Source: three-view drawing plus pictorial views. Frame: mm from the lowest corner of the part. A direction names the side the tool comes from. Coordinates: 2 decimals unless noted, no trailing zeros. Order: outer loops, then holes, each group sorted by start corner. A loop starts at its lowest first (then second) coordinate and runs counter-clockwise, first axis right, second up. Notation, with made-up numbers: (85.5, -5.5) - (110.5, -5.5) arc R22 ccw to (110.5, 16.5) - close; hole circle Ø3 at (89, 74). An arc over 180 degrees is marked (long way). One line per question, with ' | ' between items.
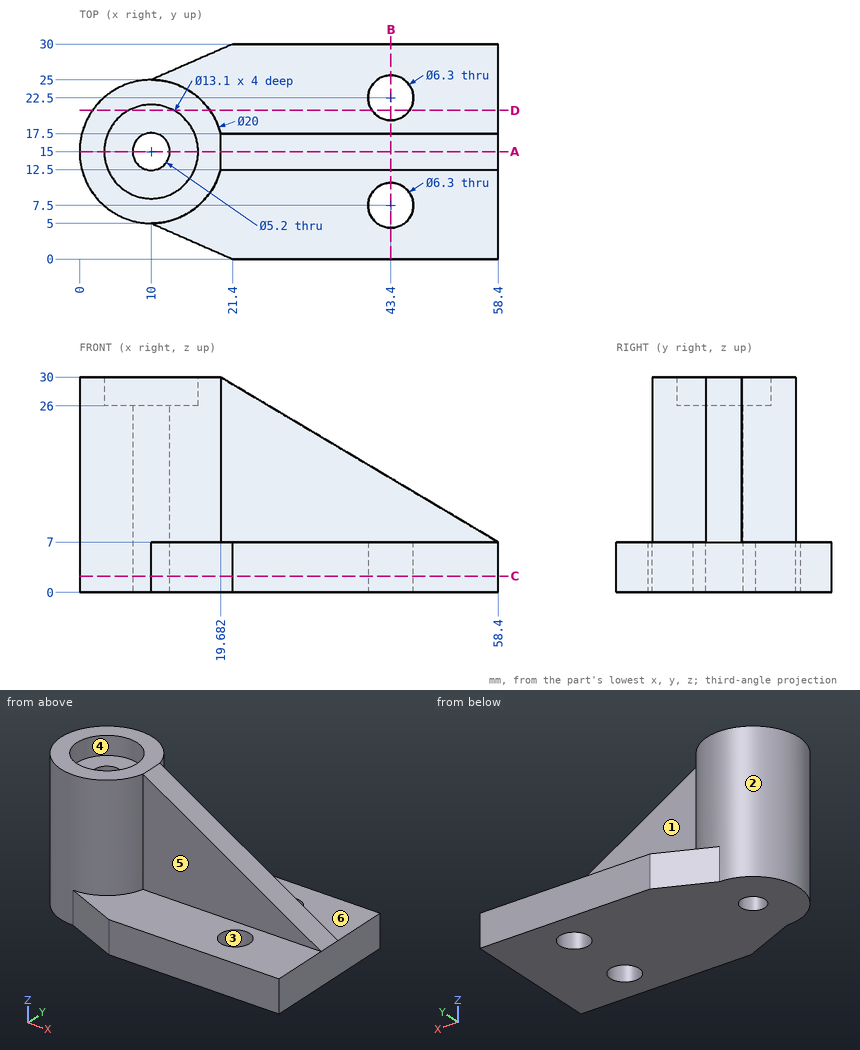
(1) Pull-direction query (X, two-part tool) for the marked faces 1, 2 and 3; classes: pulls with the +X half, pulls with the -X half, needs draft (parallel to the pull), parting line crosses it, or undercut.
Taken from the geometry:
face 1: needs draft | face 2: parting line crosses it | face 3: undercut
(2) Pin query (flat end, axial travel): P1, Ø1, axis at x = 29, y = 14, coming from the +Z side; P2, Ø5, axis at y = 21, z = 23.5, coming from the +X side; P3, Ø10, axis at x = 34, y = 3.5, coming from the +Z side. Return the tip coordinate at first contact, or that it passes through.
Taken from the geometry:
P1: stops at z = 24.76 | P2: stops at x = 19.37 | P3: stops at z = 7
(3) Cut plane A-A (y = 15). Return the cut outline in (x, z), and give its area (3 significant figures).
Taken from the geometry:
outline: (0, 0) - (7.4, 0) - (7.4, 26) - (3.45, 26) - (3.45, 30) - (0, 30) - close; (12.6, 0) - (58.4, 0) - (58.4, 7) - (19.68, 30) - (16.55, 30) - (16.55, 26) - (12.6, 26) - close | area: 1,120 mm²
(4) Material intervals for L1, parallel to Y at x = 43.4, z = 4; L2, parallel to Y at x = 10, z = 16; L3, parallel to Y at x = 19, z = 17 (1 decimal), sorted ascending. Write a range as from..to.
Taken from the geometry:
L1: y = 0..4.35, 10.65..19.35, 25.65..30 | L2: y = 5..12.4, 17.6..25 | L3: y = 10.6..19.4
(5) Set-up query: the marked faces 4, 5 and 6. Return all of +Z, -Z, +X, -X, +Y, -Y with unobstructed straight access to the full face (end or side cutting, diameter ignored); none if empty.
Taken from the geometry:
face 4: +Z | face 5: +Z, +X, -Y | face 6: +Z, +X, +Y
(6) Cut plane D-D (y = 20.75). Return the cut outline in (x, z).
Taken from the geometry:
outline: (1.82, 0) - (40.78, 0) - (40.78, 7) - (18.18, 7) - (18.18, 30) - (13.14, 30) - (13.14, 26) - (6.86, 26) - (6.86, 30) - (1.82, 30) - close; (46.02, 0) - (58.4, 0) - (58.4, 7) - (46.02, 7) - close
(7) Cut plane C-C (z = 2.25). Return the cut outline in (x, y), and give its area (3 significant figures).
Taken from the geometry:
outline: (10, 5) - (21.4, 0) - (58.4, 0) - (58.4, 30) - (21.4, 30) - (10, 25) arc R10 ccw to start; hole circle Ø5.2 at (10, 15); hole circle Ø6.3 at (43.4, 7.5); hole circle Ø6.3 at (43.4, 22.5) | area: 1,470 mm²
(8) Cut plane B-B (x = 43.4). Return the cut outline in (y, z).
Taken from the geometry:
outline: (0, 0) - (4.35, 0) - (4.35, 7) - (0, 7) - close; (10.65, 0) - (19.35, 0) - (19.35, 7) - (17.5, 7) - (17.5, 15.91) - (12.5, 15.91) - (12.5, 7) - (10.65, 7) - close; (25.65, 0) - (30, 0) - (30, 7) - (25.65, 7) - close
